Job drawing, mm, ordinate dimensions from the low corner. One solid piece. A direction names the side the tool comes from. Round coordinates to 2 decimals unless told otherwise and drop trailing zeros. Loops run counter-clockwise (first coordinate to the right, second up) from the corner with the lowest first, then second, coordinate; pieces in that order, holes last.
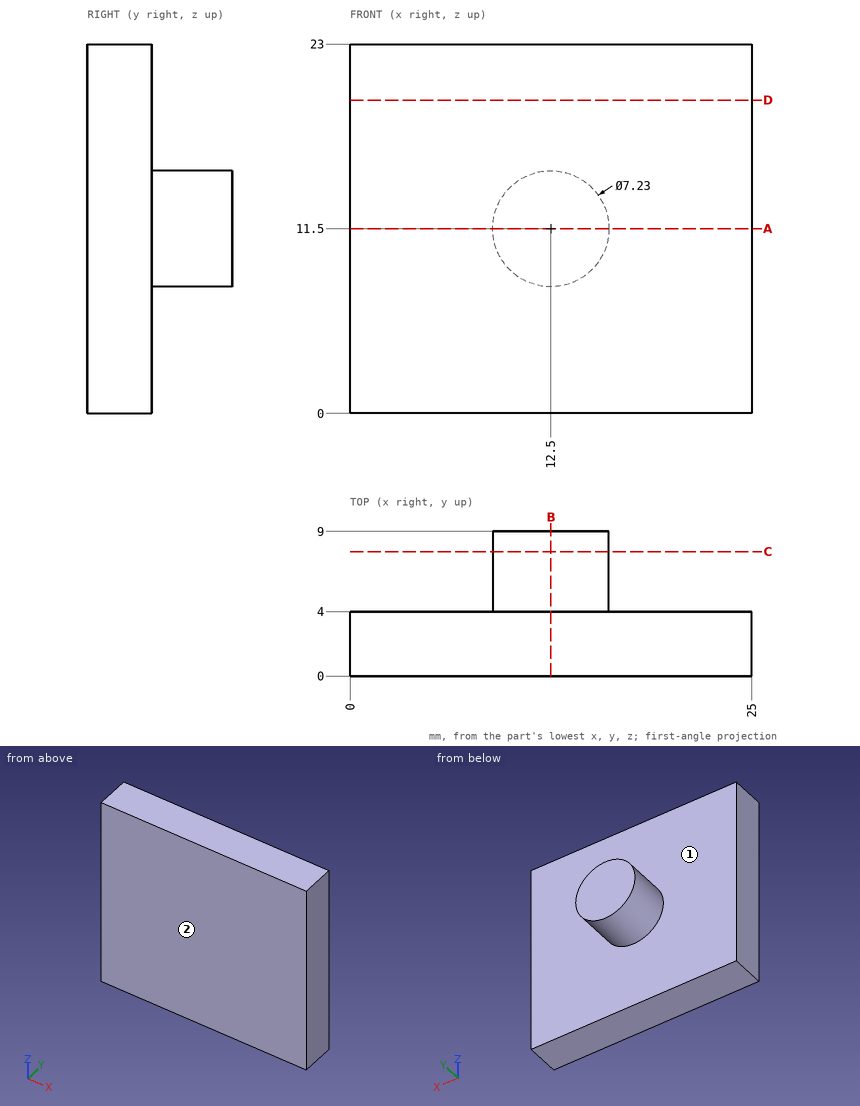
Item 1: Cut at C-C, the plane y = 7.75. Give the cut face in (x, z) (3 decimals), plus the area to 3 significant figures.
Answers follow:
outline: circle Ø7.23 at (12.5, 11.5)
area: 41.1 mm2
Item 2: Probe line 1 (Y direction, x = 3.5, z = 11.5); line 2 (Z direction, x = 9.25, y = 7.75); line 3 (Z direction, x = 14.5, y = 5). List the from-to ranges inside material, lowest first.
Answers follow:
line 1: y = 0 to 4
line 2: z = 9.92 to 13.08
line 3: z = 8.49 to 14.51
Item 3: Cut at D-D, the plane z = 19.5. Give the cut face in (x, y), plus the area to 3 significant figures.
Answers follow:
outline: (0, 0) - (25, 0) - (25, 4) - (0, 4) - close
area: 100 mm2
Item 4: Cut at B-B, the plane x = 12.5. Give the cut face in (y, z) (3 decimals), plus the area to 3 significant figures.
Answers follow:
outline: (0, 0) - (4, 0) - (4, 7.885) - (9, 7.885) - (9, 15.115) - (4, 15.115) - (4, 23) - (0, 23) - close
area: 128 mm2
Item 5: Cut at A-A, the plane z = 11.5. Give the cut face in (x, y) (3 decimals), plus the area to 3 significant figures.
Answers follow:
outline: (0, 0) - (25, 0) - (25, 4) - (16.115, 4) - (16.115, 9) - (8.885, 9) - (8.885, 4) - (0, 4) - close
area: 136 mm2
Item 6: 3-axis set-ups, long thin cutter, end or side, ignore diameter. For the marked faces 1 and 2: which of +Z, -Z, +X, -X, +Y, -Y reach the whole face in a straight line?
Answers follow:
face 1: +Y
face 2: +Z, -Z, +X, -X, -Y
